from build123d import *

# Parameters (mm, degrees)
ESQUISSE1_W             = 30
ESQUISSE1_H             = 20
BOSS_EXTRU_1_DEPTH      = 3
ESQUISSE2_R             = 3.25
ENL_V_MAT_EXTRU_1_DEPTH = 3
CONG_1_R                = 1


with BuildPart() as part:
    # Esquisse1 → Boss.-Extru.1 (new body)
    with BuildSketch(Plane.XY):
        with Locations((-5.07782823, -0.973871734)):
            Rectangle(ESQUISSE1_W, ESQUISSE1_H)
    extrude(amount=BOSS_EXTRU_1_DEPTH)

    # Esquisse2 → Enlèv. mat.-Extru.1 (cut)
    with BuildSketch(Plane.XY.offset(3)):
        with Locations((-5.07782823, -0.973871734)):
            Circle(ESQUISSE2_R)
    extrude(amount=-ENL_V_MAT_EXTRU_1_DEPTH, mode=Mode.SUBTRACT)

    # Congé1
    cong_1_edges = [part.edges().sort_by_distance(p)[0] for p in [
        (9.92217177, -0.973871734, 3),
        (-5.07782823, 9.026128266, 3),
        (-8.32782823, -0.973871734, 3),
        (-20.07782823, -0.973871734, 3),
        (-5.07782823, -10.973871734, 3),
    ]]
    fillet(cong_1_edges, radius=CONG_1_R)


solid = part.part
Here's how the part is built. I have some questions about the finished solid (model axes, mm). Give positions to 0.01 mm unless a question says otherwise; leave off trailing zeros. Order: outer loops, then holes, each group sorted by start corner. A loop starts at its lowest first (then second) coordinate and runs counter-clockwise, first axis right, second up. Notation, with made-up numbers: (48, -27.75) -> (81, -27.75) arc R7 ccw to (81, -15.75) -> close; hole circle Ø1 at (34, 64.25). An arc over 180 degrees is marked (long way). One line per item, written item: value. Start each with the question number.
1. Imagine slicing it at A-A, the plane z = 2.65. List the corners of the cut face in (x, y) for me.
2. Imagine slicing it at B-B, the plane z = 0.7. List the corners of the cut face in (x, y) for me.
3. We'd pull the mould along X, two halves only. Please class faces 1 (the face through (-19.79, -0.83, 2.7)), 2 (the face through (-7.66, -2.95, 1.01)), 3 (the face through (-5, -10.974, 1)): released by +X, released by -X, zero draft, split by the parting line, or undercut.
4. I need wall thicknesses on probe 1 along X at (y, z) = (-5.75, 2.05); probe 2 along X at (y, z) = (1, 0.7); probe 3 along X at (y, z) = (-2, 2.85). Which ranges of each line are inside material? Lowest first, please. Write a range as from..to.
Values follow:
1. outline: (-19.84, -10.73) -> (9.68, -10.73) -> (9.68, 8.79) -> (-19.84, 8.79) -> close; hole circle Ø6.98 at (-5.08, -0.97)
2. outline: (-20.08, -10.97) -> (9.92, -10.97) -> (9.92, 9.03) -> (-20.08, 9.03) -> close; hole circle Ø6.5 at (-5.08, -0.97)
3. face 1: released by -X
3. face 2: undercut
3. face 3: zero draft
4. probe 1: x = -20.08..9.92
4. probe 2: x = -20.08..-7.66, -2.5..9.92
4. probe 3: x = -19.6..-8.66, -1.5..9.45
